Read the model definition and answer for the solid it produces. Units are mm, in the model's axes. A direction names the side the tool comes from. Round coordinates to 2 decimals unless told otherwise and drop trailing zeros. Write each loop counter-clockwise with the first axis right and the second up, starting at its lowest first coordinate (ties: lowest second). Pieces come first, ordered by that corner, then holes. Notation, with made-up numbers: (-25.5, -20) - (13.5, -20) arc R25 ccw to (13.5, -1) - close; hole circle Ø1 at (5.5, -15.75). An arc over 180 degrees is marked (long way). Answer as CSV lines item,"result". Start each with the question number.
1) For a pull along Z with two mould halves and no side action, classify faces 1 (the flat face through (0, 6, -16.5)), 2 (the cylindrical face through (1.2, 6.1, 11.6)), 3 (the flat face through (-0.1, 0, -12.5)) as +Z half, -Z half, draft (parallel to the pull), parting line (faces both ways), or undercut.
2) Find section B-B on x = 0. Determine the outline of the cut face in (y, z), then the cut area to 3 significant figures.
3) Each of these flat-tipped pins is pushed along its axis until it touches: pin 1 (2 mm diameter, centred on x = -0.5, z = 2.5, fed in from -Y); pin 2 (6 mm diameter, centred on x = 5.5, z = 5.5, fed in from -Y). Where does it stop, or does it pass through?
4) Find section D-D on y = 10.5. Determine the outline of the cut face in (x, z).
5) Which of the six approach directions +Z, -Z, +X, -X, +Y, -Y give full straight-line access (tool end or side, diameter ignored) to faces 4 (the flat face through (0, 3, 6)), 5 (the flat face through (-0.1, 0, 12.3))?
6) Find section C-C on z = -10. Determine the outline of the cut face in (x, y), then the cut area to 3 significant figures.
7) Find section A-A on y = 1.5. Determine the outline of the cut face in (x, z), then the cut area to 3 significant figures.
8) Consider line 1 along Z through (x, y) = (6.5, 4.75); line 2 along X through (y, z) = (4.5, -10); line 3 along Y through (x, z) = (-5.75, -3). Determine where each line is inside the solid, lowest interval first.
from build123d import *

# Parameters (mm, degrees)
CROQUIS1_W              = 17
CROQUIS1_H              = 33
SALIENTE_EXTRUIR1_DEPTH = 12
CROQUIS2_R              = 2
CORTAR_EXTRUIR1_DEPTH   = 23.102036105
CROQUIS3_W              = 12
CROQUIS3_H              = 6.5
CORTAR_EXTRUIR2_DEPTH   = 27.55654345


with BuildPart() as part:
    # Croquis1 → Saliente-Extruir1 (new body)
    with BuildSketch(Plane(origin=(0, 0, 0), x_dir=(1, 0, 0), z_dir=(0, 1, 0))):
        Rectangle(CROQUIS1_W, CROQUIS1_H)
    extrude(amount=SALIENTE_EXTRUIR1_DEPTH)

    # Croquis2 → Cortar-Extruir1 (cut, through all)
    with BuildSketch(Plane(origin=(0, 12, 0), x_dir=(1, 0, 0), z_dir=(0, 1, 0))):
        with Locations(Location((0, 10, 0), (0, 0, 270))):
            Circle(CROQUIS2_R)
        with Locations(Location((0, -10, 0), (0, 0, 90))):
            Circle(CROQUIS2_R)
    extrude(amount=-CORTAR_EXTRUIR1_DEPTH, mode=Mode.SUBTRACT)

    # Croquis3 → Cortar-Extruir2 (cut, through all)
    with BuildSketch(Plane(origin=(8.5, 0, 0), x_dir=(0, 0, -1), z_dir=(1, 0, 0))):
        with Locations((0, 3.25)):
            Rectangle(CROQUIS3_W, CROQUIS3_H)
    extrude(amount=-CORTAR_EXTRUIR2_DEPTH, mode=Mode.SUBTRACT)


solid = part.part
Check values:
1,face 1,"-Z half"
1,face 2,"undercut"
1,face 3,"draft"
2,outline,"(0, -16.5) - (12, -16.5) - (12, -12) - (0, -12) - close; (0, -8) - (12, -8) - (12, 8) - (0, 8) - (0, 6) - (6.5, 6) - (6.5, -6) - (0, -6) - close; (0, 12) - (12, 12) - (12, 16.5) - (0, 16.5) - close"
2,area,"222 mm^2"
3,pin 1,"stops at y = 6.5"
3,pin 2,"stops at y = 0"
4,outline,"(-8.5, -16.5) - (8.5, -16.5) - (8.5, 16.5) - (-8.5, 16.5) - close; hole circle Ø4 at (0, -10); hole circle Ø4 at (0, 10)"
5,face 4,"+X, -X, -Y"
5,face 5,"+Z, -Z, +X, -X, -Y"
6,outline,"(-8.5, 0) - (-2, 0) - (-2, 12) - (-8.5, 12) - close; (2, 0) - (8.5, 0) - (8.5, 12) - (2, 12) - close"
6,area,"156 mm^2"
7,outline,"(-8.5, -16.5) - (8.5, -16.5) - (8.5, -6) - (-8.5, -6) - close; (-8.5, 6) - (8.5, 6) - (8.5, 16.5) - (-8.5, 16.5) - close; hole circle Ø4 at (0, -10); hole circle Ø4 at (0, 10)"
7,area,"332 mm^2"
8,line 1,"z = -16.5 to -6, 6 to 16.5"
8,line 2,"x = -8.5 to -2, 2 to 8.5"
8,line 3,"y = 6.5 to 12"
